Verification items for the finished model (mm, model axes). Coordinates: 2 decimals unless noted, no trailing zeros. Write each loop counter-clockwise with the first axis right and the second up, starting at its lowest first coordinate (ties: lowest second). Pieces come first, ordered by that corner, then holes. Notation, with made-up numbers: (5, 3) - (13, 3) arc R16 cw to (13, 34) - close; hole circle Ø11 at (53, 82). An arc over 180 degrees is marked (long way). Answer as CSV lines item,"result". Start each with the question number.
Autodesk Inventor part; units mm, degrees
ref_plane "YZ Plane" through (0, 0, 0) normal (1, 0, 0) x (0, 1, 0)
ref_plane "XZ Plane" through (0, 0, 0) normal (0, 1, 0) x (-1, 0, 0)
ref_plane "XY Plane" through (0, 0, 0) normal (0, 0, 1) x (1, 0, 0)
sketch "Sketch1" plane through (0, 0, 0) normal (0, 0, 1) x (1, 0, 0)
  line L0 (0, -609.6) -> (-2438.4, -609.6)
  line L1 (0, -1828.8) -> (0, 1828.8)
  line L2 (-2476.5, -609.6) -> (-2438.4, -609.6)
  line L3 (-2476.5, -609.6) -> (0, -1828.8)
  line L4 (-2476.5, -609.6) -> (-2275.2249, -609.6)
  line L5 (-2275.2249, -609.6) -> (0, -1729.7107)
  line L6 (0, -1729.7107) -> (0, -1828.8)
  point P0 (0, 0)
  dimension "d0" = 88.9
extrude "Extrusion1" add sketch "Sketch1" against normal blind 38.1 contours L5 L1 L3 L2 L0
properties part number "s48x2x4a"
1. Cross-section at B-B (y = -1148.5). Record the cut outline in (x, z), and give its area (3 significant figures).
2. Depth check by flat-ended pin: P1, Ø3, axis at y = -1484.5, z = -7, coming from the +X side; P2, Ø12, axis at x = -1557.5, z = -4, coming from the +Y side; P3, Ø5, axis at y = -1460.5, z = -16.5, coming from the +X side. Enter the tip coordinate at first touch or a pass-through.
3. Cross-section at A-A (z = -11). Record the cut outline in (x, y), and give its area (3 significant figures).
4. Scan lines: line 1 along Y through (x, z) = (-810.5, -23); line 2 along X through (y, z) = (-1217.5, -14); line 3 along X through (y, z) = (-1613.5, -25.5). Record each from-to range of solid material in increasing order. Write a range as from..to.
Completed:
1,outline,"(-1381.86, -38.1) - (-1180.58, -38.1) - (-1180.58, 0) - (-1381.86, 0) - close"
1,area,"7,670 mm2"
2,P1,"stops at x = -495.04"
2,P2,"stops at y = -959.99"
2,P3,"stops at x = -541.76"
3,outline,"(-2476.5, -609.6) - (0, -1828.8) - (0, -1729.71) - (-2275.22, -609.6) - close"
3,area,"235,000 mm2"
4,line 1,"y = -1429.78..-1330.7"
4,line 2,"x = -1241.7..-1040.43"
4,line 3,"x = -437.33..-236.05"
